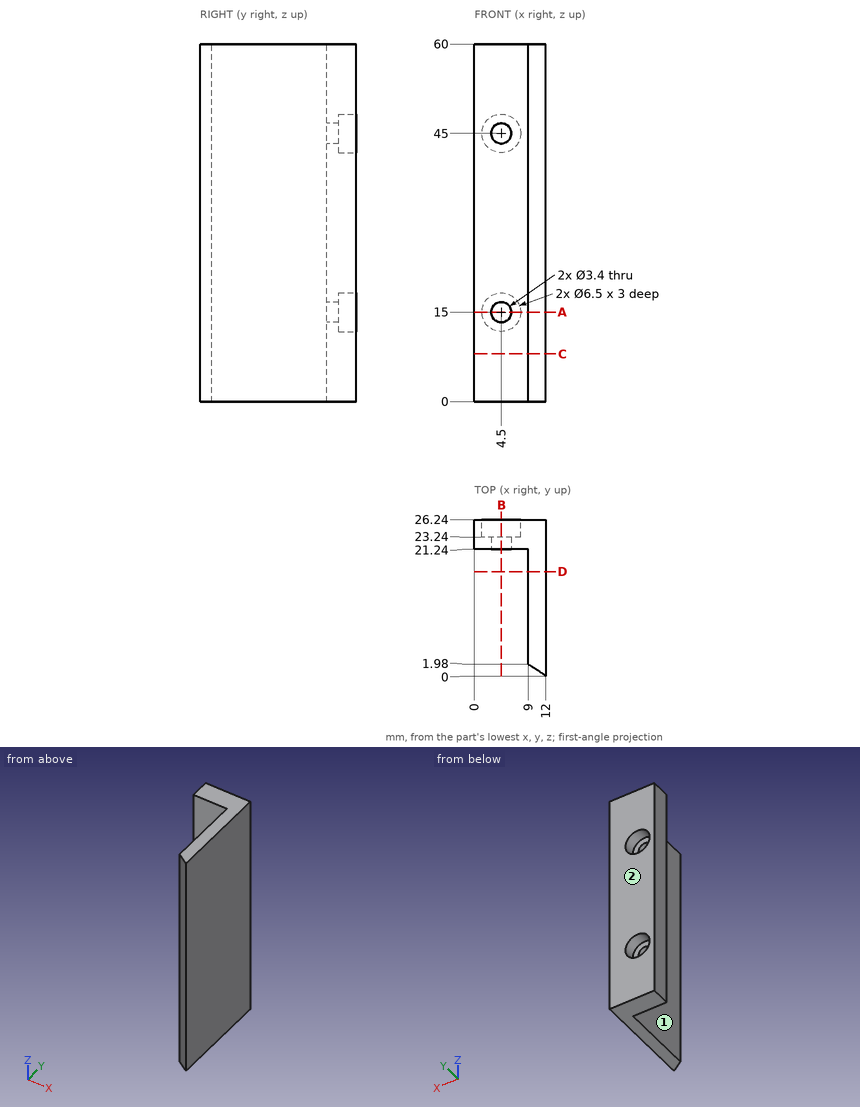
Answer from the drawing. Dimensions are ordinates in mm from the lowest x, y and z of the part. A direction names the side the tool comes from. Give positions to 0.01 mm unless a question says otherwise; leave off trailing zeros. Write each loop counter-clockwise with the first axis right and the second up, starting at its lowest first coordinate (ties: lowest second). Pieces come first, ordered by that corner, then holes.
1) Section A-A (z = 15) is taken. Write down the section's boundary in (x, y), and give its area (4 significant figures).
2) Find the intervals of material crossed by L1, parallel to Z at x = 4.5, y = 24.65; L2, parallel to X at y = 25.15, z = 15; L3, parallel to Z at x = 4.5, y = 22.35, in increasing order.
3) Section B-B (x = 4.5) is taken. Write down the section's boundary in (y, z).
4) Section D-D (y = 17.5) is taken. Write down the section's boundary in (x, z), and give its area (3 significant figures).
5) A tool of negligible diameter and unlimited length cuts with its end or side. For the marked faces 1 and 2, from which of +Z, -Z, +X, -X, +Y, -Y can it reach the whole face along a straight path? Write none if from no direction.
6) Section C-C (z = 8) is taken. Write down the section's boundary in (x, y).
7) Given P1, Ø4, axis at y = 12.5, z = 29.5, coming from the -X side; P2, Ø3, axis at x = 4, z = 13.5, coming from the +Y side; P3, Ø2, axis at x = 5, z = 52, coming from the -Y side, each flat-ended and moving along its own axis, determine where each tip first touches the part or whether it passes through.
Response:
1. outline: (0, 21.24) - (2.8, 21.24) - (2.8, 23.24) - (1.25, 23.24) - (1.25, 26.24) - (0, 26.24) - close; (6.2, 21.24) - (9, 21.24) - (9, 1.98) - (12, 0) - (12, 26.24) - (7.75, 26.24) - (7.75, 23.24) - (6.2, 23.24) - close
1. area: 94.45 mm2
2. L1: z = 0 to 11.75, 18.25 to 41.75, 48.25 to 60
2. L2: x = 0 to 1.25, 7.75 to 12
2. L3: z = 0 to 13.3, 16.7 to 43.3, 46.7 to 60
3. outline: (21.24, 0) - (26.24, 0) - (26.24, 11.75) - (23.24, 11.75) - (23.24, 13.3) - (21.24, 13.3) - close; (21.24, 16.7) - (23.24, 16.7) - (23.24, 18.25) - (26.24, 18.25) - (26.24, 41.75) - (23.24, 41.75) - (23.24, 43.3) - (21.24, 43.3) - close; (21.24, 46.7) - (23.24, 46.7) - (23.24, 48.25) - (26.24, 48.25) - (26.24, 60) - (21.24, 60) - close
4. outline: (9, 0) - (12, 0) - (12, 60) - (9, 60) - close
4. area: 180 mm2
5. face 1: +Z, -Z, -X, -Y
5. face 2: +Z, -Z, +X, -X, +Y
6. outline: (0, 21.24) - (9, 21.24) - (9, 1.98) - (12, 0) - (12, 26.24) - (0, 26.24) - close
7. P1: stops at x = 9
7. P2: stops at y = 23.24
7. P3: stops at y = 21.24
